For this review, take the finished solid that the model builds, in its own axes (mm). Give positions to 0.01 mm unless a question says otherwise; leave off trailing zeros. Order: outer loops, then holes, each group sorted by start corner. A loop starts at its lowest first (then second) coordinate and runs counter-clockwise, first axis right, second up. Notation, with made-up numbers: (8, -4) - (37, -4) arc R14 cw to (37, 10) - close; hole circle Ø1 at (-23.5, 73.25). An arc over 180 degrees is marked (long way). One line per item, written item: value.
Autodesk Inventor part; units mm, degrees
ref_plane "YZ Plane" through (0, 0, 0) normal (1, 0, 0) x (0, 1, 0)
ref_plane "XZ Plane" through (0, 0, 0) normal (0, 1, 0) x (-1, 0, 0)
ref_plane "XY Plane" through (0, 0, 0) normal (0, 0, 1) x (1, 0, 0)
sketch "Sketch1" plane through (0, 0, 0) normal (0, 1, 0) x (-1, 0, 0)
  line L0 (0, 0) -> (-69.85, 0)
  line L1 (-69.85, 0) -> (-69.85, -50.8)
  line L2 (-69.85, -50.8) -> (0, -50.8)
  line L3 (0, -50.8) -> (0, 0)
  dimension "d0" = 50.8
  dimension "d1" = 69.85
extrude "Extrusion1" add sketch "Sketch1" along normal blind 28.575
sketch "Sketch2" plane through (0, 28.575, 0) normal (0, 1, 0) x (1, 0, 0)
  line L0 (0, 0) -> (69.85, 0)
  line L1 (13.97, 0) -> (13.97, 50.8)
  line L2 (69.85, 50.8) -> (0, 50.8)
  line L3 (27.94, 50.8) -> (27.94, 0)
  line L4 (55.88, 50.8) -> (55.88, 0)
  line L5 (41.91, 50.8) -> (41.91, 0)
  line L6 (0, 50.8) -> (0, 0)
  dimension "d4" = 13.97
  dimension "d5" = 13.97
  dimension "d6" = 13.97
  dimension "d7" = 13.97
sketch "Sketch3" plane through (0, 28.575, 0) normal (0, 1, 0) x (1, 0, 0)
  line L0 (69.85, 50.8) -> (0, 50.8)
  line L1 (0, 0) -> (69.85, 0)
  line L2 (0, 50.8) -> (13.97, 50.8)
  line L3 (13.97, 50.8) -> (13.97, 0)
  line L4 (13.97, 0) -> (0, 0)
  line L5 (0, 0) -> (0, 50.8)
  dimension "d8" = 50.8
  dimension "d9" = 13.97
extrude "Extrusion2" add sketch "Sketch2" along normal blind 5 contours L6 L2 L1 L0
sketch "Sketch4" plane through (0, 0, -50.8) normal (-1, 0, 0) x (0, 0, 1)
  line L0 (0, 0) -> (0, 33.575)
  line L1 (50.8, 0) -> (50.8, 33.575)
  line L2 (0, 33.575) -> (50.8, 33.575)
  line L3 (50.8, 33.575) -> (50.8, 28.5663)
  line L4 (50.8, 28.5663) -> (0, 28.5663)
  line L5 (0, 28.5663) -> (0, 33.575)
fillet "Fillet1" radius 2 2 edges at (0, 33.575, -25.4) (13.97, 33.575, -25.4)
sketch "Sketch5" plane through (0, 28.575, 0) normal (0, 1, 0) x (1, 0, 0)
  line L0 (13.97, 50.8) -> (27.94, 50.8)
  line L1 (27.94, 50.8) -> (27.94, 0)
  line L2 (27.94, 0) -> (13.97, 0)
  line L3 (13.97, 0) -> (13.97, 50.8)
  point P0 (0, 0)
  dimension "d13" = 13.97
extrude "Extrusion3" add sketch "Sketch5" along normal blind 5
fillet "Fillet2" radius 2 2 edges at (13.97, 33.575, -25.4) (27.94, 33.575, -25.4)
sketch "Sketch6" plane through (0, 28.575, 0) normal (0, 1, 0) x (1, 0, 0)
  line L0 (27.94, 50.8) -> (27.94, 0)
  line L1 (27.94, 50.8) -> (41.91, 50.8)
  line L2 (41.91, 50.8) -> (41.91, 0)
  line L3 (41.91, 0) -> (27.94, 0)
  line L4 (27.94, 0) -> (27.94, 50.8)
  point P0 (0, 0)
  dimension "d17" = 13.97
extrude "Extrusion4" add sketch "Sketch6" along normal blind 5
fillet "Fillet3" radius 2 2 edges at (27.94, 33.575, -25.4) (41.91, 33.575, -25.4)
sketch "Sketch7" plane through (0, 28.575, 0) normal (0, 1, 0) x (1, 0, 0)
  line L0 (41.91, 0) -> (41.91, 50.8)
  line L1 (41.91, 0) -> (69.85, 0)
  line L2 (41.91, 50.8) -> (55.88, 50.8)
  line L3 (55.88, 50.8) -> (55.88, 0)
  line L4 (55.88, 0) -> (41.91, 0)
  line L5 (41.91, 0) -> (41.91, 50.8)
  point P0 (0, 0)
extrude "Extrusion5" add sketch "Sketch7" along normal blind 5
fillet "Fillet4" radius 2 2 edges at (41.91, 33.575, -25.4) (55.88, 33.575, -25.4)
sketch "Sketch8" plane through (0, 28.575, 0) normal (0, 1, 0) x (1, 0, 0)
  line L0 (55.88, 50.8) -> (55.88, 0)
  line L1 (55.88, 0) -> (69.85, 0)
  line L2 (55.88, 50.8) -> (69.85, 50.8)
  line L3 (69.85, 50.8) -> (69.85, 0)
  line L4 (69.85, 0) -> (55.88, 0)
  line L5 (55.88, 0) -> (55.88, 50.8)
  point P0 (0, 0)
extrude "Extrusion6" add sketch "Sketch8" along normal blind 5
fillet "Fillet5" radius 2 2 edges at (55.88, 33.575, -25.4) (69.85, 33.575, -25.4)
sketch "Sketch9" plane through (0, 0, 0) normal (0, -1, 0) x (1, 0, 0)
  point P0 (0, 0)
sketch "Sketch10" plane through (0, 0, 0) normal (0, -1, 0) x (1, 0, 0)
  line L0 (69.85, -50.8) -> (0, -50.8)
  line L1 (0, 0) -> (13.97, 0)
  line L2 (13.97, 0) -> (13.97, -50.8)
  line L3 (13.97, -50.8) -> (0, -50.8)
  line L4 (0, -50.8) -> (0, 0)
  dimension "d27" = 13.97
extrude "Extrusion7" add sketch "Sketch10" along normal blind 5
fillet "Fillet6" radius 2 2 edges at (0, -5, -25.4) (13.97, -5, -25.4)
sketch "Sketch11" plane through (0, 0, 0) normal (0, -1, 0) x (1, 0, 0)
  line L0 (13.97, 0) -> (13.97, -50.8)
  line L1 (27.94, -50.8) -> (25.94, -50.8)
  line L2 (13.97, 0) -> (27.94, 0)
  line L3 (27.94, 0) -> (27.94, -50.8)
  line L4 (27.94, -50.8) -> (13.97, -50.8)
  line L5 (13.97, -50.8) -> (13.97, 0)
  point P0 (0, 0)
extrude "Extrusion8" add sketch "Sketch11" along normal blind 5
fillet "Fillet7" radius 2 2 edges at (13.97, -5, -25.4) (27.94, -5, -25.4)
sketch "Sketch12" plane through (0, 0, 0) normal (0, -1, 0) x (1, 0, 0)
  line L0 (27.94, 0) -> (27.94, -50.8)
  line L1 (41.91, 0) -> (41.91, -50.8)
  line L2 (27.94, 0) -> (41.91, 0)
  line L3 (41.91, 0) -> (41.91, -50.8)
  line L4 (41.91, -50.8) -> (27.94, -50.8)
  line L5 (27.94, -50.8) -> (27.94, 0)
  point P0 (0, 0)
extrude "Extrusion9" add sketch "Sketch12" along normal blind 5
fillet "Fillet8" radius 2 2 edges at (27.94, -5, -25.4) (41.91, -5, -25.4)
sketch "Sketch13" plane through (0, 0, 0) normal (0, -1, 0) x (1, 0, 0)
  line L0 (41.91, -50.8) -> (41.91, 0)
  line L1 (69.85, -50.8) -> (41.91, -50.8)
  line L2 (41.91, 0) -> (55.88, 0)
  line L3 (55.88, 0) -> (55.88, -50.8)
  line L4 (55.88, -50.8) -> (41.91, -50.8)
  line L5 (41.91, -50.8) -> (41.91, 0)
  point P0 (0, 0)
extrude "Extrusion10" add sketch "Sketch13" along normal blind 5
fillet "Fillet9" radius 2 2 edges at (55.88, -5, -25.4) (41.91, -5, -25.4)
sketch "Sketch14" plane through (0, 0, 0) normal (0, -1, 0) x (1, 0, 0)
  line L0 (53.88, 0) -> (55.88, 0)
  line L1 (69.85, -50.8) -> (55.88, -50.8)
  line L2 (55.88, 0) -> (69.85, 0)
  line L3 (69.85, 0) -> (69.85, -50.8)
  line L4 (69.85, -50.8) -> (55.88, -50.8)
  line L5 (55.88, -50.8) -> (55.88, 0)
  point P0 (0, 0)
extrude "Extrusion11" add sketch "Sketch14" along normal blind 5
fillet "Fillet10" radius 2 2 edges at (55.88, -5, -25.4) (69.85, -5, -25.4)
sketch "Sketch15" plane through (2, 33.575, 0) normal (0, 0, 1) x (1, 0, 0)
  line L0 (-2, -2) -> (-2, -36.575)
  line L1 (-2, -19.2875) -> (67.85, -19.2875)
  line L2 (67.85, -36.575) -> (67.85, -2)
  line L3 (-2, -19.2875) -> (-2, 10.3755)
  line L4 (-2, 10.3755) -> (71.5202, 10.3755)
  line L5 (71.5202, 10.3755) -> (67.85, -19.2875)
  point P0 (-2, -33.575)
extrude "Extrusion12" cut sketch "Sketch15" against normal through all
sketch "Sketch16" plane through (69.85, -3, 0) normal (1, 0, 0) x (0, 0, -1)
  line L0 (50.8, 17.2875) -> (0, 17.2875)
  line L1 (0, 0) -> (0, 17.2875)
  line L2 (50.8, 0) -> (0, 0)
  line L3 (50.8, 0) -> (50.8, 17.2875)
  point P0 (0, 3)
extrude "Extrusion13" add sketch "Sketch16" along normal blind 13.97
ref_plane "Work Plane1" through (69.85, -3, 0) normal (1, 0, 0) x (0, 0, -1)
mirror "Mirror1" about plane through (69.85, -3, 0) normal (1, 0, 0) of "Fillet10", "Extrusion11"
properties part number "Battery"
(1) For P1, Ø8, axis at y = 6.5, z = -17.5, coming from the -X side, flat-tipped, find the tip position at first contact; note if it passes through.
Answers below:
P1: stops at x = 0
(2) Wall thickness on line 1 (Y direction, x = 27, z = -22); line 2 (Y direction, x = 13.5, z = -48): over which ranges is each line inside the solid? List them lowest first. Write a range as from..to.
Answers below:
line 1: y = -4.7..14.29
line 2: y = -4.29..14.29
(3) Take a section at B-B (x = 41). Write out the cut boundary in (y, z), then the cut area to 3 significant figures.
Answers below:
outline: (-4.68, -50.8) - (14.29, -50.8) - (14.29, 0) - (-4.68, 0) - close
area: 963 mm^2
(4) Take a section at A-A (x = 27). Write out the cut boundary in (y, z).
Answers below:
outline: (-4.7, -50.8) - (14.29, -50.8) - (14.29, 0) - (-4.7, 0) - close
(5) Draft analysis for pull direction X (two halves, no side actions). For faces 1 (the face through (41.34, -4.4, -25.76)), 2 (the face through (0.57, -4.4, -25.04)), 3 (the face through (21, -5, -25)), 4 (the face through (83.22, -4.43, -25.04)), state which applies: pulls with the +X half, pulls with the -X half, needs draft (parallel to the pull), parting line crosses it, or undercut.
Answers below:
face 1: undercut
face 2: pulls with the -X half
face 3: needs draft
face 4: pulls with the +X half
